Input: part model. Units: mm. Frame: model coordinates. Face numbers are marked on the shaded views. A direction names the side the tool comes from. Coordinates: 2 decimals unless noted, no trailing zeros. Write each loop counter-clockwise with the first axis right and the second up, starting at its lowest first coordinate (ties: lowest second). Pieces come first, ordered by that corner, then holes. Notation, with made-up numbers: (-23, -10.5) -> (-5, -10.5) arc R19 ccw to (-5, 3.5) -> close; hole circle Ø8 at (35, 36.25). An arc over 180 degrees is marked (long way). Use one line per item in the form item = value. Start each with the question number.
(1) Cut plane D-D on y = 34.5. Return the cut outline in (x, z), plus the area to 3 significant figures.
(2) Ray query, line 1 along Y through (x, z) = (-0.25, -98.5); line 2 along Z through (x, y) = (-2.75, 25); line 3 along Z through (x, y) = (-14.25, 25). Return the intervals inside material, ascending.
(3) Set-up query: the marked faces 1 and 2. Return all of +Z, -Z, +X, -X, +Y, -Y with unobstructed straight access to the full face (end or side cutting, diameter ignored); none if empty.
(4) Cut plane B-B on z = -98.5. State how many separate pieces and enclosed holes the cut face has, plus the area to 3 significant figures.
(5) First-contact query: pin 1 (1 mm diameter, centred on y = 75.5, z = -18.5, fed in from -X); pin 2 (3 mm diameter, centred on x = -9.5, y = 1, fed in from -Z); pin 3 (12 mm diameter, centred on x = -10.5, z = -68.5, fed in from +Y). Flat tips, straight axial feed; report the tip coordinate or a pass-through.
```python
from build123d import *

# Parameters (mm, degrees)
BASE_DEPTH            = 2.5
BOSS_EXTRUDE6_DEPTH   = 22
SKETCH17_W            = 12
SKETCH17_H            = 30
BOSS_EXTRUDE8_DEPTH   = 1
CUT_EXTRUDE2_REACH    = 175.139
BOSS_EXTRUDE9_DEPTH   = 24.5
SKETCH20_W            = 17
SKETCH20_H            = 8.5
CUT_EXTRUDE5_DEPTH    = 1.2
CUT_EXTRUDE6_DEPTH    = 5
SKETCH28_R            = 5
BOSS_EXTRUDE11_DEPTH  = 6
SKETCH29_R            = 3
CUT_EXTRUDE11_DEPTH   = 2
CUT_EXTRUDE12_REACH   = 175.203
SKETCH30_R            = 1.6
SKETCH31_W            = 10
SKETCH31_H            = 25
BATTERY_SUPPORT_DEPTH = 3.4
CUT_EXTRUDE9_DEPTH    = 1
CUT_EXTRUDE10_REACH   = 175.336
CUT_EXTRUDE13_DEPTH   = 1
SKETCH33_W            = 23.5
SKETCH33_H            = 0.8
CUT_EXTRUDE14_DEPTH   = 1
CHAMFER1_SIZE         = 1
CUT_EXTRUDE7_REACH    = 175.139
SKETCH23_W            = 6
SKETCH23_H            = 2.2


with BuildPart() as part:
    # Sketch1 → Base (new body)
    with BuildSketch(Plane(origin=(0, 0, 0), x_dir=(0, 0, -1), z_dir=(1, 0, 0))):
        Polygon((0, 0), (0, 77), (127, 77), (153, 51), (153, 18), (132, 0), align=None)
    extrude(amount=BASE_DEPTH)

    # Sketch11 → Boss-Extrude6 (add)
    with BuildSketch(Plane.ZY):
        Polygon((-153, 18), (-132, 0), (0, 0), (0, 77), (-127, 77), (-153, 51), align=None)
        Polygon((-150.5, 19.149837306), (-131.075189809, 2.5), (-2.5, 2.5), (-2.5, 74.5), (-125.964466094, 74.5), (-150.5, 49.964466094), align=None, mode=Mode.SUBTRACT)
    extrude(amount=BOSS_EXTRUDE6_DEPTH)

    # Sketch17 → Boss-Extrude8 (add)
    with BuildSketch(Plane(origin=(0, 77, 0), x_dir=(1, 0, 0), z_dir=(0, 1, 0))):
        with Locations((-11, 24)):
            Rectangle(SKETCH17_W, SKETCH17_H)
    extrude(amount=BOSS_EXTRUDE8_DEPTH)

    # Sketch13 → Cut-Extrude2 (cut, up to next)
    with BuildSketch(Plane(origin=(0, 78, 0), x_dir=(1, 0, 0), z_dir=(0, 1, 0)), mode=Mode.PRIVATE) as cut_extrude2_sk1:
        with BuildLine():
            Line((-22, 11.5), (-11, 11.5))
            ThreePointArc((-11, 11.5), (-8.5, 14), (-11, 16.5))
            Line((-11, 16.5), (-11, 21.5))
            ThreePointArc((-11, 21.5), (-8.5, 24), (-11, 26.5))
            Line((-11, 26.5), (-11, 31.5))
            ThreePointArc((-11, 31.5), (-8.5, 34), (-11, 36.5))
            Line((-11, 36.5), (-22, 36.5))
            Line((-22, 36.5), (-22, 11.5))
        make_face()
    cut_extrude2_tool1 = extrude(cut_extrude2_sk1.sketch, amount=-CUT_EXTRUDE2_REACH, mode=Mode.PRIVATE) & part.part
    add(cut_extrude2_tool1.solids().sort_by_distance((-15.865292, 78, -24))[0], mode=Mode.SUBTRACT)

    # Sketch19 → Boss-Extrude9 (add)
    with BuildSketch(Plane(origin=(2.5, 0, 0), x_dir=(0, 0, -1), z_dir=(1, 0, 0))):
        Polygon((127, 77), (128.697056275, 77), (140.364318164, 65.33273811), (139.515790027, 64.484209973), align=None)
    extrude(amount=-BOSS_EXTRUDE9_DEPTH)

    # Sketch20 → Cut-Extrude5 (cut)
    with BuildSketch(Plane(origin=(0, 102.848528137, -102.848528137), x_dir=(-1, 0, 0), z_dir=(0, 0.7071067811865467, -0.7071067811865485))):
        with Locations((11, -48.805339059)):
            Rectangle(SKETCH20_W, SKETCH20_H)
    extrude(amount=-CUT_EXTRUDE5_DEPTH, mode=Mode.SUBTRACT)

    # Sketch21 → Cut-Extrude6 (cut, symmetric)
    with BuildSketch(Plane(origin=(0, 102, -102), x_dir=(-1, 0, 0), z_dir=(0, 0.7071067811865478, -0.7071067811865472))):
        with BuildLine():
            Line((11, -48.005339059), (22, -48.005339059))
            Line((22, -48.005339059), (22, -53.105339059))
            Line((22, -53.105339059), (11, -53.105339059))
            ThreePointArc((11, -53.105339059), (8.45, -50.555339059), (11, -48.005339059))
        make_face()
    extrude(amount=CUT_EXTRUDE6_DEPTH, both=True, mode=Mode.SUBTRACT)

    # Sketch28 → Boss-Extrude11 (add)
    with BuildSketch(Plane(origin=(2.5, 0, 0), x_dir=(0, 0, -1), z_dir=(1, 0, 0))):
        with Locations((6.1, 70.9)):
            Circle(SKETCH28_R)
        with Locations((146.9, 44.9)):
            Circle(SKETCH28_R)
        with Locations((98.5, 6.1)):
            Circle(SKETCH28_R)
        with Locations((6.1, 6.1)):
            Circle(SKETCH28_R)
    extrude(amount=-BOSS_EXTRUDE11_DEPTH)

    # Sketch29 → Cut-Extrude11 (cut)
    with BuildSketch(Plane(origin=(2.5, 0, 0), x_dir=(0, 0, -1), z_dir=(1, 0, 0))):
        with Locations((6.1, 70.9)):
            Circle(SKETCH29_R)
        with Locations((146.9, 44.9)):
            Circle(SKETCH29_R)
        with Locations((98.5, 6.1)):
            Circle(SKETCH29_R)
        with Locations((6.1, 6.1)):
            Circle(SKETCH29_R)
    extrude(amount=-CUT_EXTRUDE11_DEPTH, mode=Mode.SUBTRACT)

    # Sketch30 → Cut-Extrude12 (cut, up to next)
    with BuildSketch(Plane(origin=(0.5, 0, 0), x_dir=(0, 0, -1), z_dir=(1, 0, 0)), mode=Mode.PRIVATE) as cut_extrude12_sk1:
        with Locations((6.1, 70.9)):
            Circle(SKETCH30_R)
    cut_extrude12_tool1 = extrude(cut_extrude12_sk1.sketch, amount=-CUT_EXTRUDE12_REACH, mode=Mode.PRIVATE) & part.part
    # Sketch30 → Cut-Extrude12 (cut, up to next)
    with BuildSketch(Plane(origin=(0.5, 0, 0), x_dir=(0, 0, -1), z_dir=(1, 0, 0)), mode=Mode.PRIVATE) as cut_extrude12_sk2:
        with Locations((6.1, 6.1)):
            Circle(SKETCH30_R)
    cut_extrude12_tool2 = extrude(cut_extrude12_sk2.sketch, amount=-CUT_EXTRUDE12_REACH, mode=Mode.PRIVATE) & part.part
    # Sketch30 → Cut-Extrude12 (cut, up to next)
    with BuildSketch(Plane(origin=(0.5, 0, 0), x_dir=(0, 0, -1), z_dir=(1, 0, 0)), mode=Mode.PRIVATE) as cut_extrude12_sk3:
        with Locations((146.9, 44.9)):
            Circle(SKETCH30_R)
    cut_extrude12_tool3 = extrude(cut_extrude12_sk3.sketch, amount=-CUT_EXTRUDE12_REACH, mode=Mode.PRIVATE) & part.part
    # Sketch30 → Cut-Extrude12 (cut, up to next)
    with BuildSketch(Plane(origin=(0.5, 0, 0), x_dir=(0, 0, -1), z_dir=(1, 0, 0)), mode=Mode.PRIVATE) as cut_extrude12_sk4:
        with Locations((98.5, 6.1)):
            Circle(SKETCH30_R)
    cut_extrude12_tool4 = extrude(cut_extrude12_sk4.sketch, amount=-CUT_EXTRUDE12_REACH, mode=Mode.PRIVATE) & part.part
    add(cut_extrude12_tool1.solids().sort_by_distance((0.5, 70.9, -6.1))[0], mode=Mode.SUBTRACT)
    add(cut_extrude12_tool2.solids().sort_by_distance((0.5, 6.1, -6.1))[0], mode=Mode.SUBTRACT)
    add(cut_extrude12_tool3.solids().sort_by_distance((0.5, 44.9, -146.9))[0], mode=Mode.SUBTRACT)
    add(cut_extrude12_tool4.solids().sort_by_distance((0.5, 6.1, -98.5))[0], mode=Mode.SUBTRACT)

    # Sketch31 → Battery_Support (add)
    with BuildSketch(Plane.ZY):
        with Locations((-9.5, 35)):
            Rectangle(SKETCH31_W, SKETCH31_H)
    extrude(amount=BATTERY_SUPPORT_DEPTH)

    # Sketch25 → Cut-Extrude9 (cut)
    with BuildSketch(Plane(origin=(2.5, 0, 0), x_dir=(0, 0, -1), z_dir=(1, 0, 0))):
        Polygon((55.5, 10.5), (132.5, 10.5), (137, 14), (137, 40), (127.5, 51), (83.5, 51), (55.5, 27), align=None)
    extrude(amount=-CUT_EXTRUDE9_DEPTH, mode=Mode.SUBTRACT)

    # Sketch26 → Cut-Extrude10 (cut, up to next)
    with BuildSketch(Plane(origin=(1.5, 0, 0), x_dir=(0, 0, -1), z_dir=(1, 0, 0)), mode=Mode.PRIVATE) as cut_extrude10_sk1:
        Polygon((57.5, 26.080130155), (57.5, 12.5), (131.8137845, 12.5), (135, 14.978167611), (135, 39.255906978), (126.584646936, 49), (84.239848152, 49), align=None)
    cut_extrude10_tool1 = extrude(cut_extrude10_sk1.sketch, amount=-CUT_EXTRUDE10_REACH, mode=Mode.PRIVATE) & part.part
    add(cut_extrude10_tool1.solids().sort_by_distance((1.5, 29.217081, -99.285701))[0], mode=Mode.SUBTRACT)

    # Sketch32 → Cut-Extrude13 (cut)
    with BuildSketch(Plane(origin=(2.5, 0, 0), x_dir=(0, 0, -1), z_dir=(1, 0, 0))):
        Polygon((144.515790027, 63.684209973), (79.121592497, 63.684209973), (51.490014195, 40), (0, 40), (0, 40.8), (51.194074935, 40.8), (78.825653236, 64.484209973), (144.515790027, 64.484209973), align=None)
    extrude(amount=-CUT_EXTRUDE13_DEPTH, mode=Mode.SUBTRACT)

    # Sketch33 → Cut-Extrude14 (cut)
    with BuildSketch(Plane.XY):
        with Locations((-10.25, 40.4)):
            Rectangle(SKETCH33_W, SKETCH33_H)
    extrude(amount=-CUT_EXTRUDE14_DEPTH, mode=Mode.SUBTRACT)

    # Chamfer1
    chamfer1_edges = [part.edges().sort_by_distance(p)[0] for p in [
        (-9.75, 40, 0),
        (2.5, 40, -25.745007098),
        (2.5, 51.842104986, -65.305803346),
        (2.5, 63.684209973, -109.718691262),
    ]]
    chamfer(chamfer1_edges, length=CHAMFER1_SIZE - 0.0001)  # a hair under: the kernel refuses the full size

    # Sketch23 → Cut-Extrude7 (cut, up to next)
    with BuildSketch(Plane.XZ, mode=Mode.PRIVATE) as cut_extrude7_sk1:
        Polygon((-5.5, -10.5), (-8, -10.5), (-14, -10.5), (-16.5, -10.5), (-16.5, -60.5), (-5.5, -60.5), align=None)
    cut_extrude7_tool1 = extrude(cut_extrude7_sk1.sketch, amount=-CUT_EXTRUDE7_REACH, mode=Mode.PRIVATE) & part.part
    # Sketch23 → Cut-Extrude7 (cut, up to next)
    with BuildSketch(Plane.XZ, mode=Mode.PRIVATE) as cut_extrude7_sk2:
        with Locations((-11, -9.4)):
            Rectangle(SKETCH23_W, SKETCH23_H)
    cut_extrude7_tool2 = extrude(cut_extrude7_sk2.sketch, amount=-CUT_EXTRUDE7_REACH, mode=Mode.PRIVATE) & part.part
    # Sketch23 → Cut-Extrude7 (cut, up to next)
    with BuildSketch(Plane.XZ, mode=Mode.PRIVATE) as cut_extrude7_sk3:
        with Locations((-11, -122.5)):
            Rectangle(SKETCH23_W, SKETCH23_H)
    cut_extrude7_tool3 = extrude(cut_extrude7_sk3.sketch, amount=-CUT_EXTRUDE7_REACH, mode=Mode.PRIVATE) & part.part
    add(cut_extrude7_tool1.solids().sort_by_distance((-11, 0, -35.5))[0], mode=Mode.SUBTRACT)
    add(cut_extrude7_tool2.solids().sort_by_distance((-11, 0, -9.4))[0], mode=Mode.SUBTRACT)
    add(cut_extrude7_tool3.solids().sort_by_distance((-11, 0, -122.5))[0], mode=Mode.SUBTRACT)


solid = part.part
```
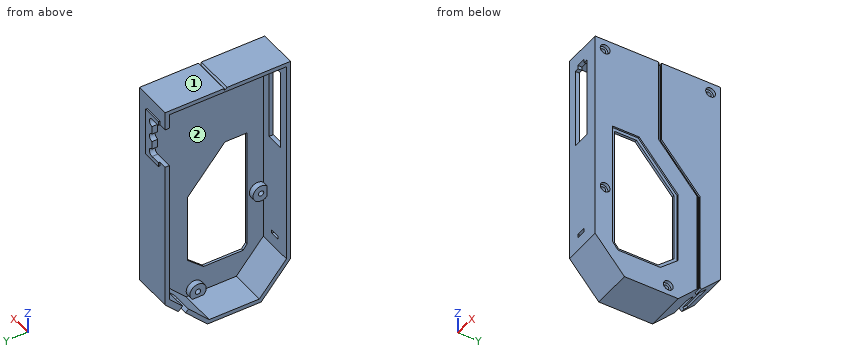
Values:
q1.outline = (-22, -153) -> (2.5, -153) -> (2.5, -137) -> (1.5, -137) -> (1.5, -135) -> (0, -135) -> (0, -150.5) -> (-22, -150.5) -> close; (-22, -2.5) -> (0, -2.5) -> (0, -4.5) -> (-3.4, -4.5) -> (-3.4, -14.5) -> (0, -14.5) -> (0, -67.32) -> (1.5, -67.32) -> (1.5, -64.25) -> (2.5, -64.25) -> (2.5, 0) -> (-22, 0) -> close
q1.area = 352 mm2
q2.line_1 = 0 to 4.5, 7.7 to 11.1, 74.5 to 77
q2.line_2 = -153 to -150.5, -14.5 to -4.5, -2.5 to 0
q2.line_3 = -153 to -150.5, -2.5 to 0
q3.face_1 = +Z, +X, -X, +Y, -Y
q3.face_2 = -X
q4.separate_pieces = 3
q4.enclosed_holes = 0
q4.area = 211 mm2
q5.pin_1 = -11
q5.pin_2 = -134.92
q5.pin_3 = 77
